Check sheet for the modelled part. Datum: model origin and axes. Units: mm. A direction names the side the tool comes from. Coordinates: 2 decimals unless noted, no trailing zeros. Write each loop counter-clockwise with the first axis right and the second up, starting at its lowest first coordinate (ties: lowest second). Pieces come first, ordered by that corner, then holes. Notation, with made-up numbers: (53.25, -2.5) - (65.25, -2.5) arc R10 cw to (65.25, 6.5) - close; hole circle Ø4 at (69, 8.25). An arc over 180 degrees is marked (long way). Answer as CSV lines item,"result". Start each with the question number.
from build123d import *

# Parameters (mm, degrees)
BOX_W     = 14
BOX_H     = 14
BOX_DEPTH = 2
FILLET_R  = 1


with BuildPart() as fillet_body:
    # Box → Box (new body)
    with BuildSketch(Plane.XY):
        with Locations((7, 7)):
            Rectangle(BOX_W, BOX_H)
    extrude(amount=BOX_DEPTH)

    # Fillet
    fillet_edges = [fillet_body.edges().sort_by_distance(p)[0] for p in [
        (0, 0, 1),
        (0, 14, 1),
        (14, 0, 1),
        (14, 14, 1),
    ]]
    fillet(fillet_edges, radius=FILLET_R)


with BuildPart() as fusion:
    # Cone → Cone (revolve)
    with BuildSketch(Plane(origin=(7, 7, 0), x_dir=(1, 0, 0), z_dir=(0, -1, 0))):
        Polygon((0, 0), (6, 0), (1, 20), (0, 20), align=None)
    revolve(axis=Axis((7, 7, 0), (0, 0, 1)))

    # Fusion: union Fillet body
    add(fillet_body.part)


solid = fusion.part
(1) Tool access check on faces 1 (the face through (13.699, 0.285, 1.014)), 2 (the face through (4, 12, 2)). Record the directions out of +Z, -Z, +X, -X, +Y, -Y that give a thin tool (end or side, any length) a straight path to the whole face; none if there is none.
(2) Material ranges on probe 1 along Z at (x, y) = (1.75, 9.5); probe 2 along Y at (x, z) = (6, 18.5); probe 3 along Y at (x, z) = (6.25, 12.5), recorded low to high. Write a range as from..to.
(3) Cross-section at C-C on z = 10.25. Record the boundary of the cut face in (x, y) (1 decimal).
(4) Cross-section at D-D on x = 12.75. Record the boundary of the cut face in (y, z), plus the area to 3 significant figures.
(5) Cross-section at A-A on x = 7. Record the boundary of the cut face in (y, z).
(6) Go/stop test with flat-tipped pins: P1, Ø8, axis at y = 2.5, z = 8.5, coming from the +X side; P2, Ø1, axis at y = 10, z = 8.5, coming from the +X side. Record where each tip stops, or that it passes through.
Checked values:
1,face 1,"+Z, -Z, +X, -Y"
1,face 2,"+Z"
2,probe 1,"0..2"
2,probe 2,"6.06..7.94"
2,probe 3,"4.22..9.78"
3,outline,"circle Ø6.9 at (7, 7)"
4,outline,"(0, 0) - (14, 0) - (14, 2) - (0, 2) - close"
4,area,"28.0 mm^2"
5,outline,"(0, 0) - (14, 0) - (14, 2) - (12.5, 2) - (8, 20) - (6, 20) - (1.5, 2) - (0, 2) - close"
6,P1,"x = 11.28"
6,P2,"x = 9.99"
